The model under review builds one solid part; all positions refer to its coordinate system, in mm. Round coordinates to 2 decimals unless told otherwise and drop trailing zeros. Write each loop counter-clockwise with the first axis right and the second up, starting at its lowest first coordinate (ties: lowest second). Pieces come first, ordered by that corner, then holes. Notation, with made-up numbers: (53.25, 84.5) - (93.25, 84.5) arc R26 cw to (93.25, 110.5) - close; hole circle Ø6 at (18.25, 69). An arc over 180 degrees is marked (long way). Return JSON: item names as keys, results as strings.
from build123d import *

# Parameters (mm, degrees)
SKETCH1_W               = 54.3999928
SKETCH1_H               = 34.798
SKETCH1_W_2             = 38.3999994
SKETCH1_H_2             = 6.849999
BOSS_EXTRUDE1_DEPTH     = 1.999996
CUT_EXTRUDE1_DEPTH      = 33.350656704
CUT_EXTRUDE1_DEPTH_BACK = 5.5500016
SKETCH2_R               = 1.8750026
BOSS_EXTRUDE2_START     = -0.2500122
SKETCH3_R               = 1.8750026
SKETCH3_R_2             = 1.2499975
BOSS_EXTRUDE2_DEPTH     = 0.2500122


with BuildPart() as part:
    # Sketch1 → Boss-Extrude1 (new body)
    with BuildSketch(Plane(origin=(0, 0, 0), x_dir=(1, 0, 0), z_dir=(0, 1, 0))):
        Rectangle(SKETCH1_W, SKETCH1_H)
        with BuildLine():
            Line((-21.2000084, -11.224006), (21.2000084, -11.224006))
            ThreePointArc((21.2000084, -11.224006), (23.3250105, -13.3490081), (21.2000084, -15.4740102))
            Line((21.2000084, -15.4740102), (-21.2000084, -15.4740102))
            ThreePointArc((-21.2000084, -15.4740102), (-23.3250105, -13.3490081), (-21.2000084, -11.224006))
        make_face(mode=Mode.SUBTRACT)
        with BuildLine():
            Line((-21.2000084, 11.224006), (21.2000084, 11.224006))
            ThreePointArc((21.2000084, 11.224006), (23.3250105, 13.3490081), (21.2000084, 15.4740102))
            Line((21.2000084, 15.4740102), (-21.2000084, 15.4740102))
            ThreePointArc((-21.2000084, 15.4740102), (-23.3250105, 13.3490081), (-21.2000084, 11.224006))
        make_face(mode=Mode.SUBTRACT)
        with Locations((-1.27e-05, 5.9702065)):
            Rectangle(SKETCH1_W_2, SKETCH1_H_2, mode=Mode.SUBTRACT)
        with Locations((-1.27e-05, -5.9702065)):
            Rectangle(SKETCH1_W_2, SKETCH1_H_2, mode=Mode.SUBTRACT)
    extrude(amount=BOSS_EXTRUDE1_DEPTH)

    # Sketch2 → Cut-Extrude1 (cut, two sides: drawn at the far end of the back side and taken through both)
    with BuildSketch(Plane(origin=(0, 1.999996, 0), x_dir=(1, 0, 0), z_dir=(0, 1, 0)).offset(-CUT_EXTRUDE1_DEPTH_BACK)):
        with Locations(Location((-24.2000278, -3.0537912, 0), (0, 0, 90))):
            Circle(SKETCH2_R)
        with Locations(Location((-24.2000278, 3.0537912, 0), (0, 0, 90))):
            Circle(SKETCH2_R)
        with Locations(Location((24.2000278, 3.0537912, 0), (0, 0, 90))):
            Circle(SKETCH2_R)
        with Locations(Location((24.2000278, -3.0537912, 0), (0, 0, 90))):
            Circle(SKETCH2_R)
    extrude(amount=CUT_EXTRUDE1_DEPTH + CUT_EXTRUDE1_DEPTH_BACK, mode=Mode.SUBTRACT)

    # Sketch3 → Boss-Extrude2 (add)
    # profile 1 of 4: a face of its own
    with BuildSketch(Plane.XZ.offset(BOSS_EXTRUDE2_START)):
        with Locations(Location((-24.2000278, 3.0537912, 0), (0, 0, 270))):
            Circle(SKETCH3_R)
        with Locations(Location((-24.2000278, 3.0537912, 0), (0, 0, 90))):
            Circle(SKETCH3_R_2, mode=Mode.SUBTRACT)
    # profile 2 of 4: a face of its own
    with BuildSketch(Plane.XZ.offset(BOSS_EXTRUDE2_START)):
        with Locations(Location((-24.2000278, -3.0537912, 0), (0, 0, 270))):
            Circle(SKETCH3_R)
        with Locations(Location((-24.2000278, -3.0537912, 0), (0, 0, 270))):
            Circle(SKETCH3_R_2, mode=Mode.SUBTRACT)
    # profile 3 of 4: a face of its own
    with BuildSketch(Plane.XZ.offset(BOSS_EXTRUDE2_START)):
        with Locations(Location((24.2000278, -3.0537912, 0), (0, 0, 270))):
            Circle(SKETCH3_R)
        with Locations(Location((24.2000278, -3.0537912, 0), (0, 0, 90))):
            Circle(SKETCH3_R_2, mode=Mode.SUBTRACT)
    # profile 4 of 4: a face of its own
    with BuildSketch(Plane.XZ.offset(BOSS_EXTRUDE2_START)):
        with Locations(Location((24.2000278, 3.0537912, 0), (0, 0, 270))):
            Circle(SKETCH3_R)
        with Locations(Location((24.2000278, 3.0537912, 0), (0, 0, 270))):
            Circle(SKETCH3_R_2, mode=Mode.SUBTRACT)
    extrude(amount=BOSS_EXTRUDE2_DEPTH)


solid = part.part
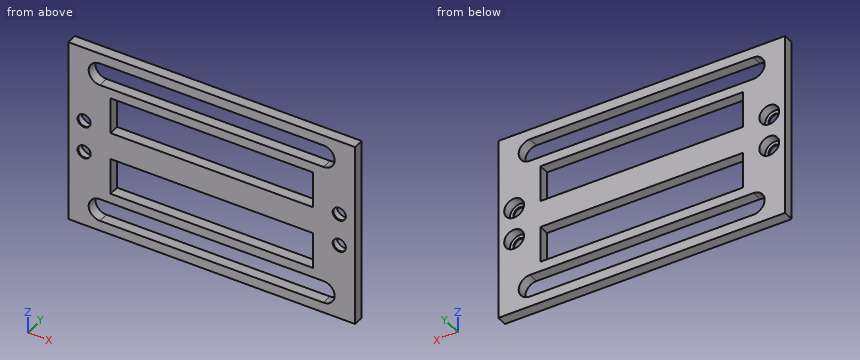
(1) Add section B-B (x = -8). Write out the cut boundary in (y, z), plus the area to 3 significant figures.
Filled in:
{"outline": "(0, -17.4) - (2, -17.4) - (2, -15.47) - (0, -15.47) - close; (0, -11.22) - (2, -11.22) - (2, -9.4) - (0, -9.4) - close; (0, -2.55) - (2, -2.55) - (2, 2.55) - (0, 2.55) - close; (0, 9.4) - (2, 9.4) - (2, 11.22) - (0, 11.22) - close; (0, 15.47) - (2, 15.47) - (2, 17.4) - (0, 17.4) - close", "area": "25.2 mm2"}
(2) Add section C-C (y = 0.6). Give the number of separate pieces and of enclosed holes in the cut face, plus the area to 3 significant figures.
Filled in:
{"separate pieces": "1", "enclosed holes": "8", "area": "934 mm2"}
(3) Add section A-A (z = 6). Write out the cut boundary in (x, y), plus the area to 3 significant figures.
Filled in:
{"outline": "(-27.2, 0) - (-19.2, 0) - (-19.2, 2) - (-27.2, 2) - close; (19.2, 0) - (27.2, 0) - (27.2, 2) - (19.2, 2) - close", "area": "32.0 mm2"}
(4) Clearance check with flat-ended pins moving along their axes: pin 1 Ø3 at (x, z) = (-24.2, -3.05) entering from +Y; pin 2 Ø3 at (x, z) = (-24.2, 3.05) entering from -Y. State where each tip first meets the part, or that it passes through.
Filled in:
{"pin 1": "stops at y = 0.25", "pin 2": "stops at y = 0"}
(5) Wall thickness on line 1 (Z direction, x = 12.5, y = 1.8); line 2 (X direction, y = 0.8, z = -7); line 3 (X direction, y = 0.6, z = 4.5): over which ranges is each line inside the solid? List them lowest first.
Filled in:
{"line 1": "z = -17.4 to -15.47, -11.22 to -9.4, -2.55 to 2.55, 9.4 to 11.22, 15.47 to 17.4", "line 2": "x = -27.2 to -19.2, 19.2 to 27.2", "line 3": "x = -27.2 to -25.39, -23.01 to -19.2, 19.2 to 23.01, 25.39 to 27.2"}
